Check sheet for the modelled part. Datum: model origin and axes. Units: mm. A direction names the side the tool comes from. Coordinates: 2 decimals unless noted, no trailing zeros. Write each loop counter-clockwise with the first axis right and the second up, starting at its lowest first coordinate (ties: lowest second). Pieces come first, ordered by that corner, then holes. Notation, with made-up numbers: M 53.25,-19 L 66.25,-19 A21 cw 66.25,-13 Z; hole C -15,-25.75 d2. An arc over 180 degrees is marked long. Answer as CSV lines item,"result". Start each with the question number.
Q1. Access from +Z, -Z, +X, -X, +Y, -Y to the whole of each face (thin tool, end or side, straight path). Record for faces 4 (the flat face through (0, 28.775, 38)), 5 (the flat face through (13.543, 0, 13)), 6 (the flat face through (0, -28.702, 57)), 7 (the flat face through (13.543, 19, 38)).
Q2. Sectioned sample at C-C, the plane y = -6.5. Record the cut outline in (x, z), then the cut area to 3 significant figures.
Q3. Sectioned sample at B-B, the plane x = 0. Count the separate pieces of the cut face and the enclosed holes in it, then the cut area to 3 significant figures.
Q4. Thickness scan on line 1 along Y through (x, z) = (0, 10); line 2 along Y through (x, z) = (-2, 40); line 3 along Y through (x, z) = (-2.5, 60). Record the ranges inside material, lowest first. Write a range as from..to.
Q5. Depth check by flat-ended pin: pin 1 Ø13.5 at (x, z) = (-4.5, 49) entering from +Y; pin 2 Ø12 at (x, y) = (0.5, 37) entering from +Z; pin 3 Ø7.5 at (x, z) = (0, 60.5) entering from -Y. Enter the tip coordinate at first touch or a pass-through.
Q6. Mould release check, pull along Y, two halves, no side actions. Record for faces 1 (the cylindrical face through (-0.523, -80.397, 12.522)), 2 (the flat face through (0, -10.414, 45)), 3 (the flat face through (-16, 1, 25.4)): pulls with the +Y half, pulls with the -Y half, needs draft (parallel to the pull), parting line crosses it, or undercut.
Q7. Sectioned sample at A-A, the plane z = 15. Record the cut outline in (x, y).
Q8. Sectioned sample at D-D, the plane y = -24.5. Record the cut outline in (x, z), then the cut area to 3 significant figures.
from build123d import *

# Parameters (mm, degrees)
F0_W      = 27.0868334974
F0_H      = 18.5560942991
F1_DEPTH  = 50.8
F0_R      = 9.3791948403
F0_R_2    = 11.0914176542
F2_DEPTH  = 25.4
F3_R      = 13.588079422
F4_DEPTH  = 25.4
F5_DEPTH  = 13.208
F6_DEPTH  = 3.302
F7_DEPTH  = 10.414
F8_R      = 13.4014797698
F9_DEPTH  = 28.702
F10_DEPTH = 10.414
F11_R     = 6.2651990724
F12_DEPTH = 36.322
F13_R     = 5.6629254321
F14_DEPTH = 82.042


with BuildPart() as f1:
    # F0 (on Top) → F1 (new body)
    with BuildSketch(Plane.XY):
        with Locations((0, -19.4966302854)):
            Rectangle(F0_W, F0_H)
    extrude(amount=F1_DEPTH)



with BuildPart() as f1b:
    # F0 (on Top) → F1, piece 2 (new body)
    with BuildSketch(Plane.XY):
        with Locations((0, 19.4966302854)):
            Rectangle(F0_W, F0_H)
    extrude(amount=F1_DEPTH)


with BuildPart() as f1_1:
    add(f1.part)

    add(f1b.part)  # F2 merges F1b
    # F0 (on Top) → F2 (join)
    with BuildSketch(Plane.XY):
        with BuildLine():
            Line((23.7966101182, -56.6057153046), (23.9485707134, -56.6057153046))
            Line((23.9485707134, -56.6057153046), (23.9485707134, 56.6057153046))
            Line((23.9485707134, 56.6057153046), (23.6905010782, 56.6057153046))
            ThreePointArc((23.6905010782, 56.6057153046), (0, 80.2962163828), (-23.6905010782, 56.6057153046))
            Line((-23.6905010782, 56.6057153046), (-23.9485707134, 56.6057153046))
            Line((-23.9485707134, 56.6057153046), (-23.9485707134, -56.6057153046))
            Line((-23.9485707134, -56.6057153046), (-23.7966101182, -56.6057153046))
            ThreePointArc((-23.7966101182, -56.6057153046), (0, -80.4023254228), (23.7966101182, -56.6057153046))
        make_face()
        with Locations((0, -56.6057153046)):
            Circle(F0_R, mode=Mode.SUBTRACT)
        Polygon((-13.5434167487, 28.7746774349), (13.5434167487, 28.7746774349), (13.5434167487, 10.2185831358), (13.5434167487, -10.2185831358), (13.5434167487, -28.7746774349), (-13.5434167487, -28.7746774349), (-13.5434167487, -10.2185831358), (-13.5434167487, 10.2185831358), align=None, mode=Mode.SUBTRACT)
        with Locations((0, 56.6057153046)):
            Circle(F0_R_2, mode=Mode.SUBTRACT)
    extrude(amount=F2_DEPTH)

    # F3 (on Front) → F4 (join)
    with BuildSketch(Plane.XZ):
        with Locations((0, 50.7737323642)):
            Circle(F3_R)
    extrude(amount=F4_DEPTH)

    # F3 (on Front) → F5 (join)
    with BuildSketch(Plane.XZ):
        with Locations((0, 50.7737323642)):
            Circle(F3_R)
    extrude(amount=F5_DEPTH)

    # F6 (add): a face of the model
    f6_faces = [f1_1.faces().sort_by_distance(p)[0] for p in [
        (0, -25.4, 56.5534391302),
    ]]
    extrude(f6_faces, amount=F6_DEPTH)

    # F7 (cut): a face of the model
    f7_faces = [f1_1.faces().sort_by_distance(p)[0] for p in [
        (0, 0, 50.7737323642),
    ]]
    extrude(f7_faces, amount=-F7_DEPTH, mode=Mode.SUBTRACT)

    # F8 (on Front) → F9 (join)
    with BuildSketch(Plane.XZ):
        with Locations((0, 50.618570298)):
            Circle(F8_R)
    extrude(amount=-F9_DEPTH)

    # F10 (cut): a face of the model
    f10_faces = [f1_1.faces().sort_by_distance(p)[0] for p in [
        (0, 0, 50.618570298),
    ]]
    extrude(f10_faces, amount=-F10_DEPTH, mode=Mode.SUBTRACT)

    # F11 (on Front) → F12 (cut)
    with BuildSketch(Plane.XZ):
        with Locations((0, 50.8907139301)):
            Circle(F11_R)
    extrude(amount=-F12_DEPTH, mode=Mode.SUBTRACT)

    # F13 (on Front) → F14 (cut)
    with BuildSketch(Plane.XZ):
        with Locations((0, 50.8907139301)):
            Circle(F13_R)
    extrude(amount=F14_DEPTH, mode=Mode.SUBTRACT)


solid = f1_1.part
Output:
1,face 4,"+Z, +X, -X, +Y"
1,face 5,"+Z, -Z"
1,face 6,"+Z, +X, -X, -Y"
1,face 7,"+Z, +X, +Y, -Y"
2,outline,"M -23.95,0 L -13.54,0 L -13.54,25.4 L -23.95,25.4 Z; M 13.54,0 L 23.95,0 L 23.95,25.4 L 13.54,25.4 Z"
2,area,"529 mm^2"
3,separate pieces,"6"
3,enclosed holes,"0"
3,area,"3,510 mm^2"
4,line 1,"y = -80.4..-65.98, -47.23..-10.22, 10.22..45.51, 67.7..80.3"
4,line 2,"y = -28.77..-10.41, 10.41..28.77"
4,line 3,"y = -28.7..-10.41, 10.41..28.7"
5,pin 1,"stops at y = 28.77"
5,pin 2,"stops at z = 25.4"
5,pin 3,"stops at y = -28.7"
6,face 1,"pulls with the -Y half"
6,face 2,"undercut"
6,face 3,"needs draft"
7,outline,"M -23.95,-56.61 L -23.8,-56.61 A23.8 ccw 23.8,-56.61 L 23.95,-56.61 L 23.95,56.61 L 23.69,56.61 A23.69 ccw -23.69,56.61 L -23.95,56.61 Z; hole M -13.54,-10.22 L 13.54,-10.22 L 13.54,10.22 L -13.54,10.22 Z; hole C 0,56.61 d22.18; hole C 0,-56.61 d18.76"
8,outline,"M -23.95,0 L 23.95,0 L 23.95,25.4 L 13.54,25.4 L 13.54,49.67 A13.59 ccw long -13.54,49.67 L -13.54,25.4 L -23.95,25.4 Z; hole C 0,50.89 d11.33"
8,area,"2,090 mm^2"
